The model under review builds one solid part; all positions refer to its coordinate system, in mm. A direction names the side the tool comes from. Coordinates: 2 decimals unless noted, no trailing zeros. Loops run counter-clockwise (first coordinate to the right, second up) from the corner with the lowest first, then second, coordinate; pieces in that order, holes last. Notation, with made-up numbers: (73.5, 53.5) - (81.5, 53.5) arc R24 ccw to (81.5, 67.5) - close; hole circle Ø3 at (-34.75, 6.5). An arc over 180 degrees is marked (long way). Use a Markdown table: item, result. Add a question column.
1) Add section B-B, the plane x = 45. Give the boundary of the cut face in (y, z), and give its area (3 significant figures).
2) For faces 4 (the flat face through (-3, 216.828, 2)), 5 (the flat face through (68, 200.53, 2)), 6 (the flat face through (-8, 150.506, 2)), 7 (the flat face through (-8, 184.514, 2)), list the 3-axis set-ups (+Z, -Z, +X, -X, +Y, -Y) from which the entire face can be reached by the end or side of a thin tool; tool diameter is ignored.
3) Add section C-C, the plane y = 146.5. Give the boundary of the cut face in (x, z), and give its area (3 significant figures).
4) The part is to be moulded in two halves that separate along Y. For faces 1 (the flat face through (-8, 192.804, 2)), 2 (the flat face through (26.317, 143, 2)), 3 (the flat face through (5, 140.522, 2)), say which applies: pulls with the +Y half, pulls with the -Y half, needs draft (parallel to the pull), parting line crosses it, or undercut.
5) To check wall thickness, follow L1, parallel to X at y = 204, z = 0.85; L2, parallel to Y at x = 42, z = 2.75; L3, parallel to Y at x = 55, z = 1.3. State the ranges of each line that lie inside material, in increasing order. Write a range as [from, to].
6) Clearance check with flat-ended pins moving along their axes: pin 1 (1.2 mm diameter, centred on y = 164, z = 2, fed in from +X); pin 2 (2 mm diameter, centred on y = 213, z = 2.5, fed in from -X); pin 3 (1.2 mm diameter, centred on x = 63.5, z = 2, fed in from +Y). State where each tip first meets the part, or that it passes through.
7) Add section A-A, the plane y = 183.5. Give the boundary of the cut face in (x, z).
```python
from build123d import *

# Parameters (mm, degrees)
BOSS_EXTRUDE1_DEPTH = 4


with BuildPart() as part:
    # Model → Boss-Extrude1 (new body)
    with BuildSketch(Plane.XY):
        Polygon((-5.997220875, 216.82832197), (1.346e-06, 216.82832197), (1.346e-06, 220.814711934), (10.301111378, 220.814711934), (10.301111378, 216.82832197), (18.026945247, 216.82832197), (18.026945247, 220.814711934), (26.31722235, 220.814711934), (26.31722235, 216.82832197), (34.007778034, 216.82832197), (34.007778034, 220.814711934), (42.333333323, 220.814711934), (42.333333323, 216.82832197), (50.023888607, 216.82832197), (50.023888607, 220.814711934), (60.325001331, 220.814711934), (60.325001331, 216.82832197), (66.322223551, 216.82832197), (66.322223551, 210.831099749), (70.308610824, 210.831099749), (70.308610824, 200.529989717), (66.322223551, 200.529989717), (66.322223551, 192.80415652), (70.308610824, 192.80415652), (70.308610824, 184.513878576), (66.322223551, 184.513878576), (66.322223551, 176.823322787), (70.308610824, 176.823322787), (70.308610824, 168.533045011), (66.322223551, 168.533045011), (66.322223551, 160.807212487), (70.308610824, 160.807212487), (70.308610824, 150.506099764), (66.322223551, 150.506099764), (66.322223551, 144.508877543), (60.325001331, 144.508877543), (60.325001331, 140.522487579), (50.023888607, 140.522487579), (50.023888607, 144.508877543), (42.333333323, 144.508877543), (42.333333323, 140.522487579), (34.007778034, 140.522487579), (34.007778034, 144.508877543), (26.31722235, 144.508877543), (26.31722235, 140.522487579), (18.026945247, 140.522487579), (18.026945247, 144.508877543), (10.301111378, 144.508877543), (10.301111378, 140.522487579), (1.346e-06, 140.522487579), (1.346e-06, 144.508877543), (-5.997220875, 144.508877543), (-5.997220875, 150.506099764), (-9.983610839, 150.506099764), (-9.983610839, 160.807212487), (-5.997220875, 160.807212487), (-5.997220875, 168.533045011), (-9.983610839, 168.533045011), (-9.983610839, 176.823322787), (-5.997220875, 176.823322787), (-5.997220875, 184.513878576), (-9.983610839, 184.513878576), (-9.983610839, 192.80415652), (-5.997220875, 192.80415652), (-5.997220875, 200.529989717), (-9.983610839, 200.529989717), (-9.983610839, 210.831099749), (-5.997220875, 210.831099749), align=None)
        with BuildLine():
            ThreePointArc((5.152925749, 201.423626349), (-2.337496568, 180.656932441), (5.167834069, 159.895621923))
            ThreePointArc((5.167834069, 159.895621923), (5.069223804, 155.557299062), (9.407474746, 155.659024168))
            ThreePointArc((9.407474746, 155.659024168), (30.162501338, 148.168599756), (50.917527931, 155.659024168))
            ThreePointArc((50.917527931, 155.659024168), (55.255778873, 155.557299062), (55.157168608, 159.895621923))
            ThreePointArc((55.157168608, 159.895621923), (62.662499244, 180.656932441), (55.172076927, 201.423626349))
            ThreePointArc((55.172076927, 201.423626349), (55.273802033, 205.761877291), (50.935479172, 205.663267026))
            ThreePointArc((50.935479172, 205.663267026), (30.162501338, 213.168599756), (9.389523504, 205.663267026))
            ThreePointArc((9.389523504, 205.663267026), (5.051200643, 205.761877291), (5.152925749, 201.423626349))
        make_face(mode=Mode.SUBTRACT)
    extrude(amount=BOSS_EXTRUDE1_DEPTH)


solid = part.part
```
From the geometry:
| question | item | result |
|---|---|---|
| 1 | outline | (144.51, 0) - (151.75, 0) - (151.75, 4) - (144.51, 4) - close; (209.58, 0) - (216.83, 0) - (216.83, 4) - (209.58, 4) - close |
| 1 | area | 58.0 mm^2 |
| 2 | face 4 | +Z, -Z, -X, +Y |
| 2 | face 5 | +Z, -Z, +X |
| 2 | face 6 | +Z, -Z, -X, -Y |
| 2 | face 7 | +Z, -Z, -X |
| 3 | outline | (-6, 0) - (66.32, 0) - (66.32, 4) - (-6, 4) - close |
| 3 | area | 289 mm^2 |
| 4 | face 1 | undercut |
| 4 | face 2 | needs draft |
| 4 | face 3 | pulls with the -Y half |
| 5 | L1 | x = [-9.98, 4.19], [56.13, 70.31] |
| 5 | L2 | y = [140.52, 150.4], [210.94, 220.81] |
| 5 | L3 | y = [140.52, 155.33], [206, 220.81] |
| 6 | pin 1 | stops at x = 66.32 |
| 6 | pin 2 | stops at x = -6 |
| 6 | pin 3 | stops at y = 216.83 |
| 7 | outline | (-6, 0) - (-2.21, 0) - (-2.21, 4) - (-6, 4) - close; (62.54, 0) - (66.32, 0) - (66.32, 4) - (62.54, 4) - close |
